Read the model definition and answer for the solid it produces. Units are mm, in the model's axes. Round coordinates to 2 decimals unless told otherwise and drop trailing zeros. Order: outer loops, then holes, each group sorted by start corner. A loop starts at its lowest first (then second) coordinate and runs counter-clockwise, first axis right, second up. Notation, with made-up numbers: (-17.75, -25.75) - (40.25, -25.75) arc R19 cw to (40.25, 10.25) - close; hole circle Ø5 at (76, 37.25). An arc over 180 degrees is marked (long way). Answer as a JSON object with one key per item and string values. Group by question number.
Q1. Given pin 1 Ø5 at (x, z) = (80, 0) entering from -Y; pin 2 Ø13.5 at (x, z) = (0, 0) entering from -Y, each flat-ended and moving along its own axis, determine where each tip first touches the part or whether it passes through.
Q2. A cutting plane is placed at B-B on z = 0. Determine the outline of the cut face in (x, y), and give its area (3 significant figures).
Q3. A cutting plane is placed at C-C on x = 80. Determine the outline of the cut face in (y, z).
Q4. Consider line 1 (Z direction, x = 0, y = -0.15); line 2 (X direction, y = -2.1, z = -1); line 3 (X direction, y = -1.4, z = 0). Determine where each line is inside the solid, lowest interval first.
Q5. The mould has two halves that part along Z. Classify faces 1 (the flat face through (-20, -2, 0)), 2 (the cylindrical face through (99.43, -2.46, 19.4)), 3 (the conical face through (4.15, -0.59, -1.72)): pulls with the +Z half, pulls with the -Z half, needs draft (parallel to the pull), parting line crosses it, or undercut.
Q6. A cutting plane is placed at A-A on y = -2.4. Determine the outline of the cut face in (x, z), and give its area (3 significant figures).
```python
from build123d import *

# Parameters (mm, degrees)
F0_R     = 4.2
F1_DEPTH = 5
F2_SIZE  = 4.7


# Not quite as in the source:
# - a feature names something its author has since deleted; it is built from what else it names


with BuildPart() as f1:
    # F0 (on Front) → F1 (new body)
    with BuildSketch(Plane.XZ):
        with BuildLine():
            Line((98, 20), (-18, 20))
            ThreePointArc((-18, 20), (-19.4142135624, 19.4142135624), (-20, 18))
            Line((-20, 18), (-20, -18))
            ThreePointArc((-20, -18), (-19.4142135624, -19.4142135624), (-18, -20))
            Line((-18, -20), (98, -20))
            ThreePointArc((98, -20), (99.4142135624, -19.4142135624), (100, -18))
            Line((100, -18), (100, 18))
            ThreePointArc((100, 18), (99.4142135624, 19.4142135624), (98, 20))
        make_face()
        Circle(F0_R, mode=Mode.SUBTRACT)
        with Locations((40, 0)):
            Circle(F0_R, mode=Mode.SUBTRACT)
        with Locations((80, 0)):
            Circle(F0_R, mode=Mode.SUBTRACT)
    extrude(amount=F1_DEPTH)

    # F2
    f2_edges = [f1.edges().sort_by_distance(p)[0] for p in [
        (-4.2, -5, 0),
        (35.8, -5, 0),
        (75.8, -5, 0),
    ]]
    chamfer(f2_edges, length=F2_SIZE)


solid = f1.part
```
Result set:
{
 "1": {"pin 1": "passes through", "pin 2": "stops at y = -2.85"},
 "2": {"outline": "(-20, -5) - (-8.9, -5) - (-4.2, -0.3) - (-4.2, 0) - (-20, 0) - close; (4.2, -0.3) - (8.9, -5) - (31.1, -5) - (35.8, -0.3) - (35.8, 0) - (4.2, 0) - close; (44.2, -0.3) - (48.9, -5) - (71.1, -5) - (75.8, -0.3) - (75.8, 0) - (44.2, 0) - close; (84.2, -0.3) - (88.9, -5) - (100, -5) - (100, 0) - (84.2, 0) - close", "area": "408 mm²"},
 "3": {"outline": "(-5, -20) - (0, -20) - (0, -4.2) - (-0.3, -4.2) - (-5, -8.9) - close; (-5, 8.9) - (-0.3, 4.2) - (0, 4.2) - (0, 20) - (-5, 20) - close"},
 "4": {"line 1": "z = -20 to -4.2, 4.2 to 20", "line 2": "x = -20 to -5.92, 5.92 to 34.08, 45.92 to 74.08, 85.92 to 100", "line 3": "x = -20 to -5.3, 5.3 to 34.7, 45.3 to 74.7, 85.3 to 100"},
 "5": {"face 1": "needs draft", "face 2": "pulls with the +Z half", "face 3": "undercut"},
 "6": {"outline": "(-20, -18) arc R2 ccw to (-18, -20) - (98, -20) arc R2 ccw to (100, -18) - (100, 18) arc R2 ccw to (98, 20) - (-18, 20) arc R2 ccw to (-20, 18) - close; hole circle Ø12.6 at (0, 0); hole circle Ø12.6 at (40, 0); hole circle Ø12.6 at (80, 0)", "area": "4,420 mm²"}
}
